Autodesk Inventor part; units mm, degrees
ref_plane "YZ Plane" through (0, 0, 0) normal (1, 0, 0) x (0, 1, 0)
ref_plane "XZ Plane" through (0, 0, 0) normal (0, 1, 0) x (-1, 0, 0)
ref_plane "XY Plane" through (0, 0, 0) normal (0, 0, 1) x (1, 0, 0)
sketch "Sketch1" plane through (0, 0, 0) normal (0, 0, 1) x (1, 0, 0)
  circle A0 centre (0, 0) radius 63.5
  circle A1 centre (0, 0) radius 35.921 construction
  line L0 (-25.4, 25.4) -> (25.4, 25.4) construction
  line L1 (25.4, 25.4) -> (25.4, -25.4) construction
  line L2 (25.4, -25.4) -> (-25.4, -25.4) construction
  line L3 (-25.4, -25.4) -> (-25.4, 25.4) construction
  circle A2 centre (-25.4, 25.4) radius 3.175
  circle A3 centre (25.4, 25.4) radius 3.175
  circle A4 centre (25.4, -25.4) radius 3.175
  circle A5 centre (-25.4, -25.4) radius 3.175
  dimension "d0" = 127
  dimension "d2" = 6.35
  dimension "d7" = 50.8
extrude "Extrusion1" add sketch "Sketch1" along normal blind 25.4
sketch "Sketch2" plane through (0, 0, 25.4) normal (0, 0, 1) x (1, 0, 0)
  circle A0 centre (0, 0) radius 63.5
extrude "Extrusion2" add sketch "Sketch2" along normal blind 127
properties part number "Motors"
The model under review builds one solid part; all positions refer to its coordinate system, in mm. A direction names the side the tool comes from. Give positions to 0.01 mm unless a question says otherwise; leave off trailing zeros. Write each loop counter-clockwise with the first axis right and the second up, starting at its lowest first coordinate (ties: lowest second). Pieces come first, ordered by that corner, then holes. Notation, with made-up numbers: (86, 64.25) -> (111, 64.25) arc R9 ccw to (111, 74.25) -> close; hole circle Ø8 at (19.5, -0.5). An arc over 180 degrees is marked (long way). Put each result on its own line as item: value.
(1) We need section D-D, the plane z = 70. Give the boundary of the cut face in (x, y), and give its area (3 significant figures).
Results are:
outline: circle Ø127 at (0, 0)
area: 12,700 mm²
(2) We need section A-A, the plane z = 20.5. Give the boundary of the cut face in (x, y) (3 decimals).
Results are:
outline: circle Ø127 at (0, 0); hole circle Ø6.35 at (-25.4, -25.4); hole circle Ø6.35 at (-25.4, 25.4); hole circle Ø6.35 at (25.4, -25.4); hole circle Ø6.35 at (25.4, 25.4)
(3) For pin 1 Ø4 at (x, y) = (-25.4, -25.4) entering from -Z; pin 2 Ø3 at (x, z) = (2.5, 78) entering from -Y; pin 3 Ø3 at (x, z) = (-44, 89.5) entering from -Y, all flat-tipped, find the tip position at first contact; note any pin that passes through.
Results are:
pin 1: z = 25.4
pin 2: y = -63.49
pin 3: y = -47.18
(4) We need section B-B, the plane y = 25.4. Give the boundary of the cut face in (x, z) (3 decimals), and give its area (3 significant figures).
Results are:
outline: (-58.199, 0) -> (-28.575, 0) -> (-28.575, 25.4) -> (-22.225, 25.4) -> (-22.225, 0) -> (22.225, 0) -> (22.225, 25.4) -> (28.575, 25.4) -> (28.575, 0) -> (58.199, 0) -> (58.199, 152.4) -> (-58.199, 152.4) -> close
area: 17,400 mm²
(5) Tool access review of faces 1 (the flat face through (-1, 1, 0)), 2 (the cylindrical face through (28.43, 24.45, 12.52)): name each direction out of +Z, -Z, +X, -X, +Y, -Y from which nothing blocks a thin tool from reaching the whole face with its end or side.
Results are:
face 1: -Z, +X, -X, +Y, -Y
face 2: -Z
(6) The part is to be moulded in two halves that separate along Y. For faces 3 (the flat face through (-25, 25, 25.4)), 4 (the cylindrical face through (-13.77, 61.99, 75.13)), 5 (the flat face through (-1, 1, 152.4)), say which applies: pulls with the +Y half, pulls with the -Y half, needs draft (parallel to the pull), parting line crosses it, or undercut.
Results are:
face 3: undercut
face 4: parting line crosses it
face 5: needs draft
(7) To check wall thickness, follow probe 1 along Y at (x, z) = (-25, 18); probe 2 along Y at (x, z) = (0, 145.5). State the ranges of each line that lie inside material, in increasing order. Write a range as from..to.
Results are:
probe 1: -58.37..-28.55, -22.25..22.25, 28.55..58.37
probe 2: -63.5..63.5
